Work out the finished part from the listing and answer in its coordinate system (mm). A direction names the side the tool comes from. Coordinates: 2 decimals unless noted, no trailing zeros. Write each loop counter-clockwise with the first axis right and the second up, starting at its lowest first coordinate (ties: lowest second). Pieces come first, ordered by that corner, then holes. Notation, with made-up numbers: (9, 12.5) - (57, 12.5) arc R16 ccw to (57, 28.5) - close; hole circle Ø11 at (-3.75, 38.5). An arc over 180 degrees is marked (long way). One line per item, written item: value.
Autodesk Inventor part; units mm, degrees
ref_plane "Plano de trabajo1" through (-24.7048, 62, 56.9407) normal (0, 0, 1) x (1, 0, 0)
ref_plane "Plano de trabajo3" through (-24.7048, 62, 1.9407) normal (0, 0, 1) x (1, 0, 0)
ref_plane "Plano de trabajo4" through (-24.7048, 62, -48.0593) normal (0, 0, 1) x (1, 0, 0)
sketch "Boceto1" plane through (0, 0, 0) normal (0, 1, 0) x (-1, 0, 0)
  line L0 (43.6381, 98.6893) -> (-16.3619, 98.6893)
  line L1 (-16.3619, 98.6893) -> (-16.3619, -111.3107)
  line L2 (-16.3619, -111.3107) -> (43.6381, -111.3107)
  line L3 (43.6381, -111.3107) -> (43.6381, 98.6893)
  point P0 (0, 0)
  dimension "d0" = 210
  dimension "d1" = 60
extrude "Extrusión1" add sketch "Boceto1" along normal blind 20
sketch "Boceto2" plane through (0, 20, 0) normal (0, 1, 0) x (1, 0, 0)
  line L0 (-38.9219, -88.6893) -> (7.0781, -88.6893)
  line L1 (7.0781, -88.6893) -> (7.0781, -73.6893)
  line L2 (7.0781, -73.6893) -> (-38.9219, -73.6893)
  line L3 (-38.9219, -73.6893) -> (-38.9219, -88.6893)
  line L4 (-38.9219, -43.6893) -> (7.0781, -43.6893)
  line L5 (7.0781, -43.6893) -> (7.0781, -13.6893)
  line L6 (7.0781, -13.6893) -> (-38.9219, -13.6893)
  line L7 (-38.9219, -13.6893) -> (-38.9219, -43.6893)
  line L8 (-38.9219, 9.3107) -> (7.0781, 9.3107)
  line L9 (7.0781, 9.3107) -> (7.0781, 39.3107)
  line L10 (7.0781, 39.3107) -> (-38.9219, 39.3107)
  line L11 (-38.9219, 39.3107) -> (-38.9219, 9.3107)
  line L12 (-38.9219, 61.3107) -> (7.0781, 61.3107)
  line L13 (7.0781, 61.3107) -> (7.0781, 91.3107)
  line L14 (7.0781, 91.3107) -> (-38.9219, 91.3107)
  line L15 (-38.9219, 91.3107) -> (-38.9219, 61.3107)
  line L16 (-43.6381, -98.6893) -> (16.3619, -98.6893)
  line L17 (16.3619, 111.3107) -> (-43.6381, 111.3107)
  point P0 (0, 0)
  dimension "d6" = 15
  dimension "d7" = 30
  dimension "d8" = 46
  dimension "d9" = 46
  dimension "d10" = 30
  dimension "d11" = 46
  dimension "d12" = 30
  dimension "d13" = 46
  dimension "d14" = 10
  dimension "d15" = 20
  dimension "d16" = 30
  dimension "d17" = 23
  dimension "d18" = 22
extrude "Extrusión2" add sketch "Boceto2" along normal blind 42
sketch "Boceto3" plane through (0, 62, 0) normal (0, 1, 0) x (1, 0, 0)
  line L0 (-4.7048, -21.9668) -> (-24.7048, -21.9668)
  line L1 (-24.7048, -21.9668) -> (-24.7048, -36.9668)
  line L2 (-24.7048, -36.9668) -> (-4.7048, -36.9668)
  line L3 (-4.7048, -36.9668) -> (-4.7048, -21.9668)
  line L4 (-24.7048, 15.3623) -> (-4.7048, 15.3623)
  line L5 (-4.7048, 15.3623) -> (-4.7048, 30.3623)
  line L6 (-4.7048, 30.3623) -> (-24.7048, 30.3623)
  line L7 (-24.7048, 30.3623) -> (-24.7048, 15.3623)
  line L8 (-24.7048, 69.8642) -> (-4.7048, 69.8642)
  line L9 (-4.7048, 69.8642) -> (-4.7048, 84.8642)
  line L10 (-4.7048, 84.8642) -> (-24.7048, 84.8642)
  line L11 (-24.7048, 84.8642) -> (-24.7048, 69.8642)
  line L12 (-24.7048, -86.9407) -> (-4.7048, -86.9407)
  line L13 (-4.7048, -86.9407) -> (-4.7048, -76.9407)
  line L14 (-4.7048, -76.9407) -> (-24.7048, -76.9407)
  line L15 (-24.7048, -76.9407) -> (-24.7048, -86.9407)
  point P0 (0, 0)
  dimension "d19" = 20
  dimension "d20" = 15
  dimension "d21" = 20
  dimension "d22" = 15
  dimension "d23" = 15
  dimension "d24" = 20
  dimension "d25" = 20
  dimension "d26" = 10
  dimension "d31" = 0
extrude "Extrusión3" add sketch "Boceto3" along normal blind 18
sketch "Sketch16" plane through (7.0781, 20, -91.3107) normal (0, 0, -1) x (-1, 0, 0)
  line L0 (-9.2838, 0) -> (50.7162, 0)
  line L1 (4.75, 36) -> (41.25, 36)
  line L2 (41.25, 36) -> (41.25, 0)
  line L3 (41.25, 0) -> (4.75, 0)
  line L4 (4.75, 0) -> (4.75, 36)
  line L5 (0, 42) -> (46, 42)
  point P0 (7.0781, -20)
  point P1 (23, 42)
  point P2 (23, 36)
  point P3 (4.75, 0)
  dimension "d57" = 36.5
  dimension "d58" = 36
extrude "Extrusion8" cut sketch "Sketch16" against normal up to surface (135 mm away)
sketch "Boceto4" plane through (-4.7048, 62, -84.8642) normal (0, 0, -1) x (-1, 0, 0)
  circle A0 centre (9.6513, 12.486) radius 5.5025
  point P0 (-4.7048, -62)
extrude "Extrusión4" add sketch "Boceto4" against normal blind 170
ref_plane "Plano de trabajo1" through (-24.7048, 62, 56.9407) normal (0, 0, 1) x (1, 0, 0)
sketch "Boceto6" plane through (-24.7048, 62, 56.9407) normal (0, 0, 1) x (1, 0, 0)
  circle A0 centre (10.3487, 12.486) radius 5.5025
  circle A1 centre (10.3487, 12.486) radius 25
  point P0 (24.7048, -62)
  point P1 (41.0667, -62)
  dimension "d33" = 74.486
  dimension "d34" = 25
extrude "Extrusión5" add sketch "Boceto6" along normal blind 5 contours A0 | A1
ref_plane "Plano de trabajo3" through (-24.7048, 62, 1.9407) normal (0, 0, 1) x (1, 0, 0)
ref_plane "Plano de trabajo4" through (-24.7048, 62, -48.0593) normal (0, 0, 1) x (1, 0, 0)
sketch "Boceto7" plane through (-24.7048, 62, 1.9407) normal (0, 0, 1) x (1, 0, 0)
  circle A0 centre (10.3487, 12.486) radius 25
  circle A1 centre (10.3487, 12.486) radius 20
  point P0 (24.7048, -62)
extrude "Extrusión6" add sketch "Boceto7" along normal blind 5 contours A0 | A1
sketch "Boceto8" plane through (-24.7048, 62, -48.0593) normal (0, 0, 1) x (1, 0, 0)
  circle A0 centre (10.3487, 12.486) radius 25
  circle A1 centre (10.3487, 12.486) radius 20
  point P0 (24.7048, -62)
  dimension "d48" = 50
extrude "Extrusión7" add sketch "Boceto8" along normal blind 5 contours A0 | A1
ref_plane "Plano de trabajo5" through (-14.3562, 74.486, 59.4407) normal (0, 0, -1) x (-1, 0, 0)
sketch "Boceto10" plane through (-14.3562, 74.486, 59.4407) normal (0, 0, -1) x (-1, 0, 0)
  line L0 (-2.688, 19.6173) -> (2.312, 19.6173)
  line L1 (2.312, 19.6173) -> (2.312, -1.3827)
  line L2 (2.312, -1.3827) -> (-2.688, -1.3827)
  line L3 (-2.688, -1.3827) -> (-2.688, 19.6173)
  line L4 (-30.7181, -74.486) -> (29.2819, -74.486)
  point P0 (-14.3562, -74.486)
  dimension "d43" = 21
  dimension "d46" = 5
revolve "Revolución1" add sketch "Boceto10" angle 360 about axis through (-11.6681, 94.1034, 59.4407) along (-1, 0, 0)
sketch "Boceto11" plane through (-14.3562, 74.486, 59.4407) normal (0, 0, -1) x (-1, 0, 0)
  point P0 (-14.3562, -74.486)
ref_plane "Plano de trabajo6" through (-22.9219, 20, 88.6893) normal (1, 0, 0) x (0, 0, -1)
sketch "Boceto14" plane through (-13.6381, 102.3503, 6.9407) normal (0, 0, 1) x (1, 0, 0)
  line L0 (-3.0387, -8.6715) -> (1.9613, -8.6715)
  line L1 (1.9613, -8.6715) -> (1.9613, -29.6715)
  line L2 (1.9613, -29.6715) -> (-3.0387, -29.6715)
  line L3 (-3.0387, -29.6715) -> (-3.0387, -8.6715)
  line L4 (-30.7181, -74.486) -> (29.2819, -74.486)
  point P0 (-14.3562, -74.486)
  dimension "d51" = 21
  dimension "d52" = 5
revolve "Revolución2" add sketch "Boceto14" angle 360 about axis through (-16.6768, 93.6788, 6.9407) along (-1, 0, 0)
sketch "Boceto15" plane through (-23.9868, 103.3042, -48.0593) normal (0, 0, 1) x (1, 0, 0)
  line L0 (7.4215, -9.5056) -> (12.4215, -9.5056)
  line L1 (12.4215, -9.5056) -> (12.4215, -30.5056)
  line L2 (12.4215, -30.5056) -> (7.4215, -30.5056)
  line L3 (7.4215, -30.5056) -> (7.4215, -9.5056)
  line L4 (-30.7181, -74.486) -> (29.2819, -74.486)
  point P0 (-14.3562, -74.486)
  dimension "d54" = 21
  dimension "d55" = 5
revolve "Revolución3" add sketch "Boceto15" angle 360 about axis through (-16.5652, 93.7986, -48.0593) along (-1, 0, 0)
sketch "Sketch17" plane through (-24.7048, 62, 86.9407) normal (0, 0, 1) x (1, 0, 0)
  circle A0 centre (10.3487, 12.486) radius 5.5025
  circle A1 centre (10.3487, 12.486) radius 1.25
  point P0 (24.7048, -62)
  dimension "d61" = 2.5
extrude "Extrusion9" cut sketch "Sketch17" against normal up to next contours A1
Item 1: Section A-A, the plane y = 43 is taken. Determine the outline of the cut face in (x, z), then the cut area to 4 significant figures.
Evaluation:
outline: (-38.92, -91.31) - (-34.17, -91.31) - (-34.17, -61.31) - (-38.92, -61.31) - close; (-38.92, -39.31) - (-34.17, -39.31) - (-34.17, -9.31) - (-38.92, -9.31) - close; (-38.92, 13.69) - (-34.17, 13.69) - (-34.17, 43.69) - (-38.92, 43.69) - close; (-38.92, 73.69) - (7.08, 73.69) - (7.08, 88.69) - (-38.92, 88.69) - close; (2.33, -91.31) - (7.08, -91.31) - (7.08, -61.31) - (2.33, -61.31) - close; (2.33, -39.31) - (7.08, -39.31) - (7.08, -9.31) - (2.33, -9.31) - close; (2.33, 13.69) - (7.08, 13.69) - (7.08, 43.69) - (2.33, 43.69) - close
area: 1,545 mm2
Item 2: Determine the mould class of faces 5 (the face through (-13, 0, -5)), 6 (the face through (-38.922, 41, -25)), 7 (the face through (2.328, 38, -25)) for opening direction Y: +Y half, -Y half, draft (parallel to the pull), parting line (faces both ways), or undercut.
Evaluation:
face 5: -Y half
face 6: draft
face 7: undercut
Item 3: Consider probe 1 along Z at (x, y) = (-25.5, 93.5); probe 2 along Y at (x, z) = (-29.5, 43.5); probe 3 along Y at (x, z) = (-16, -31). Determine where each line is inside the solid, lowest interval first.
Evaluation:
probe 1: z = -48.06 to -43.06, 1.94 to 6.94, 56.94 to 61.94
probe 2: y = 0 to 20, 56 to 62
probe 3: y = 0 to 20, 56 to 62, 69.23 to 79.74, 81.55 to 106.05
Item 4: Section B-B, the plane z = 10.5 is taken. Give the number of separate pieces and of enclosed holes in the cut face, then the cut area to 3 significant figures.
Evaluation:
separate pieces: 2
enclosed holes: 1
area: 1,460 mm2
Item 5: Which of the six approach directions +Z, -Z, +X, -X, +Y, -Y give full straight-line access (tool end or side, diameter ignored) to faces 1 (the face through (-16.895, 69.604, 46.814)), 2 (the face through (-38.922, 41, -77)), 3 (the face through (7.078, 41, 81)), 4 (the face through (2.328, 38, 28))?
Evaluation:
face 1: none
face 2: +Z, -Z, -X, +Y
face 3: +Z, -Z, +X, +Y
face 4: -Z
Item 6: Given pin 1 (12.5 mm diameter, centred on x = -5.5, y = 38, fed in from -Z); pin 2 (12 mm diameter, centred on x = -14.5, y = 48, fed in from -Z); pin 3 (5 mm diameter, centred on y = 27, z = -84, fed in from -X), each flat-ended and moving along its own axis, determine where each tip first touches the part or whether it passes through.
Evaluation:
pin 1: stops at z = 73.69
pin 2: stops at z = -48.06
pin 3: stops at x = -38.92
